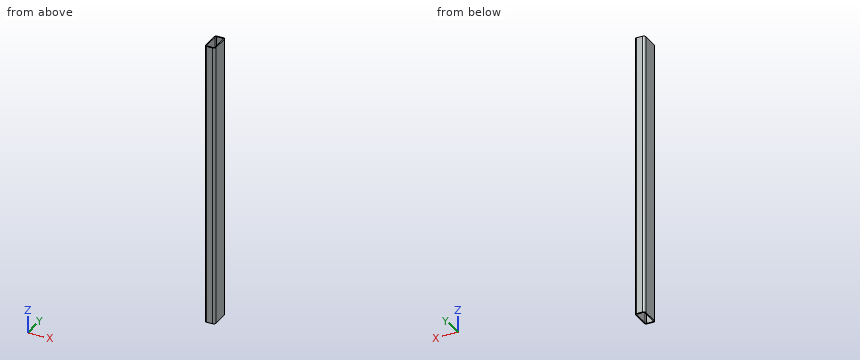
Autodesk Inventor part; units mm, degrees
ref_plane "Start Plane" through (0, 0, 20) normal (0, 0, 1) x (1, 0, 0)
ref_plane "End Plane" through (0, 0, 580) normal (0, 0, 1) x (1, 0, 0)
ref_plane "Work Plane4" through (-390, 276, 580) normal (0, 0, 1) x (1, 0, 0)
ref_plane "Start Plane" through (0, 0, 20) normal (0, 0, 1) x (1, 0, 0)
ref_plane "End Plane" through (0, 0, 580) normal (0, 0, 1) x (1, 0, 0)
sketch "Sketch" plane through (0, 0, 0) normal (0, 0, 1) x (1, 0, 0)
  line L0 (-10, -16) -> (-10, 16)
  line L1 (-6, 20) -> (6, 20)
  line L2 (10, 16) -> (10, -16)
  line L3 (6, -20) -> (-6, -20)
  arc A0 (-10, -16) -> (-6, -20) centre (-6, -16) ccw
  arc A1 (10, 16) -> (6, 20) centre (6, 16) ccw
  arc A2 (-6, 20) -> (-10, 16) centre (-6, 16) ccw
  arc A3 (6, -20) -> (10, -16) centre (6, -16) ccw
  arc A4 (-6, 18) -> (-8, 16) centre (-6, 16) ccw
  line L4 (-6, 18) -> (6, 18)
  arc A5 (8, 16) -> (6, 18) centre (6, 16) ccw
  line L5 (8, 16) -> (8, -16)
  arc A6 (6, -18) -> (8, -16) centre (6, -16) ccw
  line L6 (6, -18) -> (-6, -18)
  arc A7 (-8, -16) -> (-6, -18) centre (-6, -16) ccw
  line L7 (-8, -16) -> (-8, 16)
  line L8 (0, 29.1598) -> (0, -29.1598) construction
  line L9 (-15.1598, 0) -> (15.1598, 0) construction
  dimension "d7" = 4
  dimension "d9" = 20
  dimension "d11" = 40
  dimension "d12" = 2
  dimension "d15" = 10
  dimension "d16" = 20
extrude "Body" add sketch "Sketch" along normal up to surface (560 mm away) from surface at 20
sketch "Sketch3" plane through (0, 0, 0) normal (0, 0, 1) x (1, 0, 0)
  line L0 (0, 0) -> (10, 0)
ref_plane "Work Plane3" through (0, 0, 0) normal (0, -1, 0) x (1, 0, 0)
ref_plane "Work Plane4" through (-390, 276, 580) normal (0, 0, 1) x (1, 0, 0)
split "Split1" plane through (-390, 276, 580) removes the side toward (0, 0, 1)
ref_plane "Work Plane5" through (-480, 244, 20) normal (0, 0, -1) x (-1, 0, 0)
split "Split2" plane through (-480, 244, 20) removes the side toward (0, 0, -1)
sketch "Sketch4" plane through (0, 0, 0) normal (0, -1, 0) x (1, 0, 0)
  line L0 (-2, 20) -> (12, 20)
  line L1 (-2, 580) -> (12, 580)
  dimension "d18" = 560
equation "\"d7\" = G_IR"
equation "\"d9\" = G_W"
equation "\"d11\" = G_H"
equation "\"d12\" = G_T"
equation "\"d15\" = 0.5 * d9"
equation "\"d16\" = 0.5 * d11"
equation "\"d3\" = G_L"
equation "\"G_W\" = 20"
equation "\"G_H\" = 40"
equation "\"G_T\" = 2"
equation "\"G_IR\" = 4"
equation "\"G_L\" = d18"
properties part number "ISO 10799-2 - 40x20x2 - 560" material "Steel, Mild"
Design review of the part built by this model. Coordinates are the model's own, in mm. Round coordinates to 2 decimals unless told otherwise and drop trailing zeros. Order: outer loops, then holes, each group sorted by start corner. A loop starts at its lowest first (then second) coordinate and runs counter-clockwise, first axis right, second up. Notation, with made-up numbers: (-38, 44) - (17, 44) arc R22 ccw to (17, 60) - close; hole circle Ø10 at (54.5, 33.5). An arc over 180 degrees is marked (long way). Return JSON: item names as keys, results as strings.
Q1. Consider section C-C on y = 7.5. Write out the cut boundary in (x, z).
Computed values:
{"outline": "(-10, 20) - (-8, 20) - (-8, 580) - (-10, 580) - close; (8, 20) - (10, 20) - (10, 580) - (8, 580) - close"}
Q2. Consider section B-B on x = -1. Write out the cut boundary in (y, z), plus the area to 3 significant figures.
Computed values:
{"outline": "(-20, 20) - (-18, 20) - (-18, 580) - (-20, 580) - close; (18, 20) - (20, 20) - (20, 580) - (18, 580) - close", "area": "2,240 mm2"}
Q3. Wall thickness on L1, parallel to X at y = -7.5, z = 417.5; L2, parallel to Y at x = 0.75, z = 58; L3, parallel to X at y = 17.5, z = 66: over which ranges is each line inside the solid? List them lowest first. Write a range as [from, to].
Computed values:
{"L1": "x = [-10, -8], [8, 10]", "L2": "y = [-20, -18], [18, 20]", "L3": "x = [-9.71, -7.32], [7.32, 9.71]"}
Q4. Consider section A-A on z = 465.5. Write out the cut boundary in (x, y).
Computed values:
{"outline": "(-10, -16) arc R4 ccw to (-6, -20) - (6, -20) arc R4 ccw to (10, -16) - (10, 16) arc R4 ccw to (6, 20) - (-6, 20) arc R4 ccw to (-10, 16) - close; hole (-8, -16) arc R2 ccw to (-6, -18) - (6, -18) arc R2 ccw to (8, -16) - (8, 16) arc R2 ccw to (6, 18) - (-6, 18) arc R2 ccw to (-8, 16) - close"}
Q5. For pin 1 Ø8 at (x, y) = (2, -6.5) entering from -Z, flat-tipped, find the tip position at first contact; note if it passes through.
Computed values:
{"pin 1": "passes through"}
